```python
from build123d import *

# Parameters (mm, degrees)
F0_R     = 43.18
F0_R_2   = 12.7
F1_DEPTH = 19.05
F2_SIZE2 = 0.3402954744
F2_SIZE  = 1.27
F4_D     = 3.4544
F4_DEPTH = 11.43
F4_TIP   = 1.0378064612
F6_D     = 3.4544
F6_DEPTH = 15.24
F6_TIP   = 1.0378064612
F8_D     = 4.4958


with BuildPart() as f1:
    # F0 (on Top) → F1 (new body)
    with BuildSketch(Plane.XY):
        Circle(F0_R)
        Circle(F0_R_2, mode=Mode.SUBTRACT)
    extrude(amount=F1_DEPTH)

    # F2
    f2_edges = [f1.edges().sort_by_distance(p)[0] for p in [
        (-12.7, 0, 19.05),
        (-12.7, 0, 0),
    ]]
    f2_side = f1.faces().sort_by_distance((-12.7, 0, 9.525))[0]
    chamfer(f2_edges, length=F2_SIZE, length2=F2_SIZE2, reference=f2_side)

    # F4
    with Locations(Plane(origin=(0, 0, 0), x_dir=(1, 0, 0), z_dir=(0, 0, -1))):
        with Locations((0, -17.78), (-17.78, 0), (0, 17.78), (17.78, 0)):
            Hole(F4_D / 2, depth=F4_DEPTH)
            with Locations((0, 0, -(F4_DEPTH + F4_TIP / 2))):  # 118° drill point
                Cone(0, F4_D / 2, F4_TIP, mode=Mode.SUBTRACT)

    # F6
    with Locations(Plane.XY.offset(19.05)):
        with Locations((35, 0), (0, -35), (-35, 0), (0, 35)):
            Hole(F6_D / 2, depth=F6_DEPTH)
            with Locations((0, 0, -(F6_DEPTH + F6_TIP / 2))):  # 118° drill point
                Cone(0, F6_D / 2, F6_TIP, mode=Mode.SUBTRACT)

    # F8 (through all)
    with Locations(Plane.XY.offset(19.05)):
        with Locations((24.7487373415, -24.7487373415), (-24.7487373415, -24.7487373415), (-24.7487373415, 24.7487373415), (24.7487373415, 24.7487373415)):
            Hole(F8_D / 2)


solid = f1.part
```
The model under review builds one solid part; all positions refer to its coordinate system, in mm. A direction names the side the tool comes from. Round coordinates to 2 decimals unless told otherwise and drop trailing zeros. Write each loop counter-clockwise with the first axis right and the second up, starting at its lowest first coordinate (ties: lowest second). Pieces come first, ordered by that corner, then holes. Notation, with made-up numbers: M 70,85 L 115,85 A10 cw 115,92 Z; hole C 77,39.5 d11. An arc over 180 degrees is marked long. Use CSV: the item, a comma, the result in double quotes. Start each with the question number.
(1) Tool access review of faces 1 (the face through (-24.261, -26.943, 9.392)), 2 (the face through (0.4, -16.1, 5.8)), 3 (the face through (0.374, -36.686, 11.323)): name each direction out of +Z, -Z, +X, -X, +Y, -Y from which nothing blocks a thin tool from reaching the whole face with its end or side.
(2) We need section B-B, the plane x = -15. State the section outline as (y, z) points.
(3) The part is to be moulded in two halves that separate along X. For faces 4 (the face through (18.057, 0.115, 12.288)), 5 (the face through (-31.83, 29.18, 9.39)), 6 (the face through (9, 10, 0)), 7 (the face through (-0.22, 35.2, 2.95)), say which applies: +X half, -X half, draft (parallel to the pull), parting line (faces both ways), or undercut.
(4) We need section C-C, the plane y = 30. State the section outline as (x, z) points, then the cut area to 3 significant figures.
(5) Clearance check with flat-ended pins moving along their axes: P1, Ø3, axis at x = 11.5, z = 7.5, coming from the +Y side; P2, Ø4, axis at x = -8.5, z = 12, coming from the +Y side; P3, Ø10, axis at y = -19, z = 13, coming from the +X side. State where each tip first meets the part, or that it passes through.
(6) For line 1 along Y through (x, z) = (0, 15.5); line 2 along Y through (x, z) = (0, 5.75); line 3 along Y through (x, z) = (0, 2.5), list the stretches that pass through material, from the lowest coordinate up.
(7) We need section A-A, the plane z = 16.5. State how many separate pieces and enclosed holes the cut face has, then the cut area to 3 significant figures.
Findings:
1,face 1,"+Z, -Z"
1,face 2,"-Z"
1,face 3,"+Z"
2,outline,"M -40.49,0 L 40.49,0 L 40.49,19.05 L -40.49,19.05 Z"
3,face 4,"undercut"
3,face 5,"parting line"
3,face 6,"draft"
3,face 7,"undercut"
4,outline,"M -31.06,0 L 31.06,0 L 31.06,19.05 L -31.06,19.05 Z"
4,area,"1,180 mm^2"
5,P1,"y = 42.01"
5,P2,"y = 42.69"
5,P3,"x = 40.85"
6,line 1,"-43.18 to -36.73, -33.27 to -12.7, 12.7 to 33.27, 36.73 to 43.18"
6,line 2,"-43.18 to -36.73, -33.27 to -19.51, -16.05 to -12.7, 12.7 to 16.05, 19.51 to 33.27, 36.73 to 43.18"
6,line 3,"-43.18 to -19.51, -16.05 to -12.7, 12.7 to 16.05, 19.51 to 43.18"
7,separate pieces,"1"
7,enclosed holes,"9"
7,area,"5,250 mm^2"
